Design review of the part built by this model. Coordinates are the model's own, in mm. Face numbers are marked on the shaded views. Coordinates: 2 decimals unless noted, no trailing zeros. Loops run counter-clockwise (first coordinate to the right, second up) from the corner with the lowest first, then second, coordinate; pieces in that order, holes last. Notation, with made-up numbers: (26.5, -23) -> (76.5, -23) arc R22 ccw to (76.5, 16) -> close; hole circle Ø1 at (30, -22). An arc over 180 degrees is marked (long way). Answer in a Markdown table with one row per item.
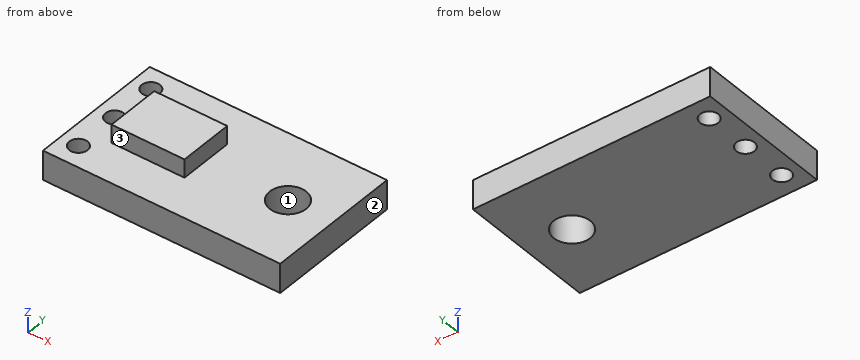
```python
from build123d import *

# Parameters (mm, degrees)
F0_W     = 13
F0_H     = 7.5
F0_R     = 0.5
F0_W_2   = 4
F0_H_2   = 3
F0_R_2   = 1
F1_DEPTH = 1.6
F2_DEPTH = 1


with BuildPart() as f1:
    # F0 (on Top) → F1 (new body)
    with BuildSketch(Plane.XY):
        Rectangle(F0_W, F0_H)
        with Locations((-5.5, -2.54)):
            Circle(F0_R, mode=Mode.SUBTRACT)
        with Locations((-5.5, 0)):
            Circle(F0_R, mode=Mode.SUBTRACT)
        with Locations((-2.5, 0)):
            Rectangle(F0_W_2, F0_H_2, mode=Mode.SUBTRACT)
        with Locations((-5.5, 2.54)):
            Circle(F0_R, mode=Mode.SUBTRACT)
        with Locations((4, 0)):
            Circle(F0_R_2, mode=Mode.SUBTRACT)
        with Locations((-2.5, 0)):
            Rectangle(F0_W_2, F0_H_2)
    extrude(amount=-F1_DEPTH)

    # F0 (on Top) → F2 (join)
    with BuildSketch(Plane.XY):
        with Locations((-2.5, 0)):
            Rectangle(F0_W_2, F0_H_2)
    extrude(amount=F2_DEPTH)


solid = f1.part
```
(1) To check wall thickness, follow probe 1 along Y at (x, z) = (-5.5, -0.8); probe 2 along Y at (x, z) = (4, -0.7); probe 3 along X at (y, z) = (2.5, -0.05). State the ranges of each line that lie inside material, in increasing order.
Evaluation:
| item | result |
|---|---|
| probe 1 | y = -3.75 to -3.04, -2.04 to -0.5, 0.5 to 2.04, 3.04 to 3.75 |
| probe 2 | y = -3.75 to -1, 1 to 3.75 |
| probe 3 | x = -6.5 to -6, -5 to 6.5 |
(2) Take a section at A-A on y = 0. Give the boundary of the cut face in (x, z), and give its area (3 significant figures).
Evaluation:
| item | result |
|---|---|
| outline | (-6.5, -1.6) -> (-6, -1.6) -> (-6, 0) -> (-6.5, 0) -> close; (-5, -1.6) -> (3, -1.6) -> (3, 0) -> (-0.5, 0) -> (-0.5, 1) -> (-4.5, 1) -> (-4.5, 0) -> (-5, 0) -> close; (5, -1.6) -> (6.5, -1.6) -> (6.5, 0) -> (5, 0) -> close |
| area | 20.0 mm² |
(3) Take a section at B-B on y = -2.54. Give the boundary of the cut face in (x, z), and give its area (3 significant figures).
Evaluation:
| item | result |
|---|---|
| outline | (-6.5, -1.6) -> (-6, -1.6) -> (-6, 0) -> (-6.5, 0) -> close; (-5, -1.6) -> (6.5, -1.6) -> (6.5, 0) -> (-5, 0) -> close |
| area | 19.2 mm² |
(4) Draft analysis for pull direction X (two halves, no side actions). For the marked faces 1, 2 and 3, state which applies: pulls with the +X half, pulls with the -X half, needs draft (parallel to the pull), parting line crosses it, or undercut.
Evaluation:
| item | result |
|---|---|
| face 1 | undercut |
| face 2 | pulls with the +X half |
| face 3 | needs draft |
(5) Take a section at D-D on x = -5.5. Give the boundary of the cut face in (y, z).
Evaluation:
| item | result |
|---|---|
| outline | (-3.75, -1.6) -> (-3.04, -1.6) -> (-3.04, 0) -> (-3.75, 0) -> close; (-2.04, -1.6) -> (-0.5, -1.6) -> (-0.5, 0) -> (-2.04, 0) -> close; (0.5, -1.6) -> (2.04, -1.6) -> (2.04, 0) -> (0.5, 0) -> close; (3.04, -1.6) -> (3.75, -1.6) -> (3.75, 0) -> (3.04, 0) -> close |
(6) Take a section at C-C on x = 4. Give the boundary of the cut face in (y, z), and give its area (3 significant figures).
Evaluation:
| item | result |
|---|---|
| outline | (-3.75, -1.6) -> (-1, -1.6) -> (-1, 0) -> (-3.75, 0) -> close; (1, -1.6) -> (3.75, -1.6) -> (3.75, 0) -> (1, 0) -> close |
| area | 8.80 mm² |
(7) For pin 1 (0.5 mm diameter, centred on x = -3.5, z = 0.5, fed in from -Y); pin 2 (0.5 mm diameter, centred on y = -0.5, z = 0.5, fed in from -X); pin 3 (0.8 mm diameter, centred on x = -1.5, z = 0.5, fed in from +Y), all flat-tipped, find the tip position at first contact; note any pin that passes through.
Evaluation:
| item | result |
|---|---|
| pin 1 | stops at y = -1.5 |
| pin 2 | stops at x = -4.5 |
| pin 3 | stops at y = 1.5 |
